```python
from build123d import *

# Parameters (mm, degrees)
F0_R     = 5.232212
F1_DEPTH = 34.036
F2_SIZE  = 5.08
F3_W     = 7.82259
F3_H     = 3.568198
F4_DEPTH = 25.4


with BuildPart() as f1:
    # F0 (on Top) → F1 (new body)
    with BuildSketch(Plane.XY):
        Circle(F0_R)
    extrude(amount=F1_DEPTH)

    # F2
    f2_edges = [f1.edges().sort_by_distance(p)[0] for p in [
        (-5.232212, 0, 34.036),
    ]]
    chamfer(f2_edges, length=F2_SIZE)

    # F3 (on Front) → F4 (cut)
    with BuildSketch(Plane.XZ):
        with Locations((0, 24.497494)):
            Rectangle(F3_W, F3_H)
    extrude(amount=-F4_DEPTH, mode=Mode.SUBTRACT)


solid = f1.part
```
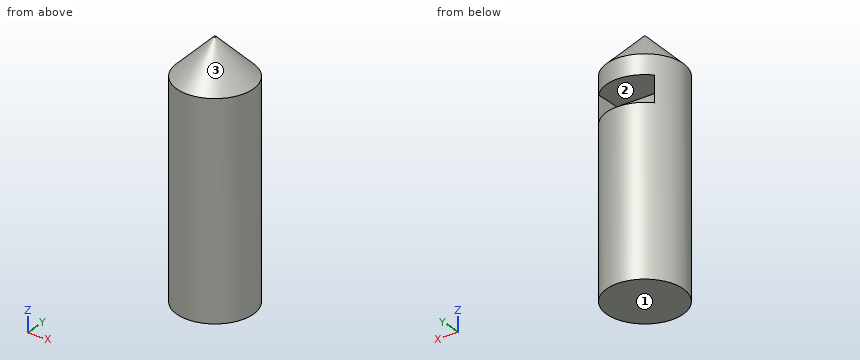
Verification items for the finished model (mm, model axes). Face numbers are marked on the shaded views. Coordinates: 2 decimals unless noted, no trailing zeros. Loops run counter-clockwise (first coordinate to the right, second up) from the corner with the lowest first, then second, coordinate; pieces in that order, holes last. Notation, with made-up numbers: (87, -31.75) -> (132, -31.75) arc R16 cw to (132, -3.75) -> close; hole circle Ø1 at (-4, 61). An arc over 180 degrees is marked (long way). Answer in a Markdown table with one row per item.
1) Scan lines: line 1 along Y through (x, z) = (0.25, 19); line 2 along Z through (x, y) = (1.25, 3.25); line 3 along Z through (x, y) = (1.5, 2.25). Record each from-to range of solid material in increasing order. Write a range as from..to.
The answers:
| item | result |
|---|---|
| line 1 | y = -5.23..5.23 |
| line 2 | z = 0..22.71, 26.28..30.71 |
| line 3 | z = 0..22.71, 26.28..31.48 |
2) Draft check along Z on the marked faces 1, 2 and 3. Enter one of: released by +Z, released by -Z, zero draft, split by the parting line, or undercut.
The answers:
| item | result |
|---|---|
| face 1 | released by -Z |
| face 2 | undercut |
| face 3 | released by +Z |
3) Section check A-A (z = 19). Record the cut outline in (x, y), and give its area (3 significant figures).
The answers:
| item | result |
|---|---|
| outline | circle Ø10.46 at (0, 0) |
| area | 86.0 mm2 |
4) Section check B-B (z = 31). Record the cut outline in (x, y), and give its area (3 significant figures).
The answers:
| item | result |
|---|---|
| outline | circle Ø6.38 at (0, 0) |
| area | 31.9 mm2 |
5) Depth check by flat-ended pin: P1, Ø1.5, axis at x = 4, z = 11.5, coming from the +Y side; P2, Ø1, axis at y = 2.5, z = 25.5, coming from the -X side; P3, Ø1, axis at x = -1, y = -2, coming from the +Z side. Enter the tip coordinate at first touch or a pass-through.
The answers:
| item | result |
|---|---|
| P1 | stops at y = 4.1 |
| P2 | stops at x = -4.83 |
| P3 | stops at z = 32.45 |
